For this review, take the finished solid that the model builds, in its own axes (mm). A direction names the side the tool comes from. Give positions to 0.01 mm unless a question says otherwise; leave off trailing zeros. Loops run counter-clockwise (first coordinate to the right, second up) from the corner with the lowest first, then second, coordinate; pieces in that order, holes last.
```python
from build123d import *

# Parameters (mm, degrees)
EXTRUDE_1_DEPTH = 3
EXTRUDE_2_DEPTH = 6


with BuildPart() as part:
    # 스케치1 → 보스-돌출1 (new body)
    with BuildSketch(Plane(origin=(0, 0, 0), x_dir=(1, 0, 0), z_dir=(0, 1, 0))):
        with BuildLine():
            Line((-26.05, 7.55), (-20.71714266, 7.55))
            ThreePointArc((-20.71714266, 7.55), (22.05, 0), (-20.71714266, -7.55))
            Line((-20.71714266, -7.55), (-26.05, -7.55))
            Line((-26.05, -7.55), (-26.05, 7.55))
        make_face()
    extrude(amount=EXTRUDE_1_DEPTH)

    # 스케치2 → 보스-돌출2 (add)
    with BuildSketch(Plane(origin=(0, 3, 0), x_dir=(1, 0, 0), z_dir=(0, 1, 0))):
        with BuildLine():
            Line((-26.05, 7.55), (-26.05, -7.55))
            Line((-26.05, -7.55), (-20.71714266, -7.55))
            ThreePointArc((-20.71714266, -7.55), (22.05, 0), (-20.71714266, 7.55))
            Line((-20.71714266, 7.55), (-26.05, 7.55))
        make_face()
        with BuildLine():
            Line((-19.077473627, 5.3), (-23.8, 5.3))
            Line((-23.8, 5.3), (-23.8, -5.3))
            Line((-23.8, -5.3), (-19.077473627, -5.3))
            ThreePointArc((-19.077473627, -5.3), (19.8, 0), (-19.077473627, 5.3))
        make_face(mode=Mode.SUBTRACT)
    extrude(amount=EXTRUDE_2_DEPTH)


solid = part.part
```
Q1. Consider section A-A on y = 4.5. Give the boundary of the cut face in (x, z), plus the area to 3 significant figures.
Answers:
outline: (-26.05, -7.55) - (-20.72, -7.55) arc R22.05 ccw (long way) to (-20.72, 7.55) - (-26.05, 7.55) - close; hole (-23.8, -5.3) - (-19.08, -5.3) arc R19.8 ccw (long way) to (-19.08, 5.3) - (-23.8, 5.3) - close
area: 318 mm2
Q2. Mouldability with a two-part tool opening along X and no side actions: class faces 5 (the flat face through (-9, 9, 18)), 6 (the flat face through (-26.05, 4, 0)), 7 (the cylindrical face through (19.784, 5.958, 0.796)) as +X half, -X half, draft (parallel to the pull), parting line (faces both ways), or undercut.
Answers:
face 5: draft
face 6: -X half
face 7: undercut
Q3. For probe 1 along Z at (x, y) = (0, 5.65); probe 2 along X at (y, z) = (7.5, -15.5); probe 3 along Z at (x, y) = (-14, 5.5), list the stretches that pass through material, from the lowest coordinate up.
Answers:
probe 1: z = -22.05 to -19.8, 19.8 to 22.05
probe 2: x = -15.68 to -12.32, 12.32 to 15.68
probe 3: z = -17.04 to -14, 14 to 17.04
Q4. Machinability: for faces 1 (the flat face through (-23, 4, 7.55)), 2 (the flat face through (-21, 6, -5.3)), 3 (the flat face through (-2, 0, 0)), 4 (the flat face through (-23, 4, -7.55)), which of the approach directions +Z, -Z, +X, -X, +Y, -Y give a long, thin tool a straight path to every point of the face, cutting with its end or side? Answer none if there is none.
Answers:
face 1: +Z, -X, +Y, -Y
face 2: +Y
face 3: +Z, -Z, +X, -X, -Y
face 4: -Z, -X, +Y, -Y
Q5. Consider section B-B on x = 0. Give the boundary of the cut face in (y, z).
Answers:
outline: (0, -22.05) - (9, -22.05) - (9, -19.8) - (3, -19.8) - (3, 19.8) - (9, 19.8) - (9, 22.05) - (0, 22.05) - close
Q6. For pin 1 Ø12 at (x, z) = (4.5, -0.5) entering from +Y; pin 2 Ø1.8 at (y, z) = (6, 2) entering from +X; pin 3 Ø1.6 at (x, y) = (-23.5, 3) entering from +Z, all flat-tipped, find the tip position at first contact; note any pin that passes through.
Answers:
pin 1: stops at y = 3
pin 2: stops at x = 22.02
pin 3: stops at z = 7.55
Q7. Consider section C-C on z = 0. Give the boundary of the cut face in (x, y).
Answers:
outline: (-26.05, 0) - (22.05, 0) - (22.05, 9) - (19.8, 9) - (19.8, 3) - (-23.8, 3) - (-23.8, 9) - (-26.05, 9) - close
Q8. Consider section D-D on y = 1.5. Give the boundary of the cut face in (x, z), plus the area to 3 significant figures.
Answers:
outline: (-26.05, -7.55) - (-20.72, -7.55) arc R22.05 ccw (long way) to (-20.72, 7.55) - (-26.05, 7.55) - close
area: 1,590 mm2
